Source: CAD feature listing. Evaluate the final solid. Frame: model axes, mm. A direction names the side the tool comes from. Round coordinates to 2 decimals unless told otherwise and drop trailing zeros. Loops run counter-clockwise (first coordinate to the right, second up) from the corner with the lowest first, then second, coordinate; pieces in that order, holes last. Notation, with made-up numbers: (79, 61) -> (90, 61) arc R14 ccw to (90, 71) -> close; hole circle Ø11 at (40, 89.5). An arc over 180 degrees is marked (long way). Put each result on its own line as item: value. Start each with the question number.
1. Draft query along Y for faces 4 (the cylindrical face through (-6.11, -7.46, 7.23)), 5 (the cylindrical face through (6.11, -0.31, 13.79)), 6 (the flat face through (0, -4, 1.219)). Return one class per face: pulls with the +Y half, pulls with the -Y half, needs draft (parallel to the pull), parting line crosses it, or undercut.
2. Cut plane B-B (z = 11.43). Return the cut outline in (x, y), then the cut area to 3 significant figures.
3. Cut plane D-D (z = 2). Return the cut outline in (x, y).
4. Set-up query: faces 1 (the flat face through (6.13, 7.06, 8.58)), 2 (the flat face through (6, 7.366, 4)), 3 (the cylindrical face through (5.967, -1.458, 0.724)). Return all of +Z, -Z, +X, -X, +Y, -Y with unobstructed straight access to the full face (end or side cutting, diameter ignored); none if empty.
5. Cut plane C-C (y = -3.75). Return the cut outline in (x, z), then the cut area to 3 significant figures.
6. Material intervals for L1, parallel to X at y = 2.5, z = 13; L2, parallel to Z at x = 4, y = -0.75; L3, parallel to Y at x = -6.1, z = 11.43, sorted ascending.
7. Contact query for flat-ended pins moving along their axis: pin 1 (5 mm diameter, centred on x = -2.5, y = -4, fed in from +Z); pin 2 (4 mm diameter, centred on x = -2, y = -3, fed in from +Z); pin 3 (1 mm diameter, centred on x = 6, z = 3.5, fed in from +Y). Output: stop coordinate, or through.
8. Cut plane A-A (z = 5.75). Return the cut outline in (x, y).
```python
from build123d import *

# Parameters (mm, degrees)
F1_DEPTH = 12.7
F2_R     = 2.38125
F3_DEPTH = 25.4
F5_DEPTH = 12.7


with BuildPart() as f1:
    # F0 (on Front) → F1 (new body, symmetric)
    with BuildSketch(Plane.XZ):
        with BuildLine():
            ThreePointArc((-6.731, 2.54), (-5.987051, 0.743949), (-4.191, 0))
            Line((-4.191, 0), (4.191, 0))
            ThreePointArc((4.191, 0), (5.987051, 0.743949), (6.731, 2.54))
            Line((6.731, 2.54), (6.731, 25.4))
            Line((6.731, 25.4), (5.5118, 25.4))
            Line((5.5118, 25.4), (5.5118, 2.54))
            ThreePointArc((5.5118, 2.54), (5.124947, 1.606053), (4.191, 1.2192))
            Line((4.191, 1.2192), (-4.191, 1.2192))
            ThreePointArc((-4.191, 1.2192), (-5.124947, 1.606053), (-5.5118, 2.54))
            Line((-5.5118, 2.54), (-5.5118, 25.4))
            Line((-5.5118, 25.4), (-6.731, 25.4))
            Line((-6.731, 25.4), (-6.731, 2.54))
        make_face()
    extrude(amount=F1_DEPTH, both=True)

    # F2 (on Right) → F3 (intersect, symmetric)
    with BuildSketch(Plane.YZ):
        with BuildLine():
            Line((-10.756956, 3.640789), (-8.382, 0))
            Line((-8.382, 0), (4.826, 0))
            ThreePointArc((4.826, 0), (5.572779, 1.793221), (7.366, 2.54))
            Line((7.366, 2.54), (7.366, 5.003639))
            Line((7.366, 5.003639), (4.896118, 6.262106))
            ThreePointArc((4.896118, 6.262106), (4.230106, 8.311882), (6.279882, 8.977894))
            Line((6.279882, 8.977894), (7.852802, 8.176451))
            Line((7.852802, 8.176451), (8.298947, 9.052059))
            ThreePointArc((8.298947, 9.052059), (8.373581, 9.510956), (8.167681, 9.927802))
            Line((8.167681, 9.927802), (3.468643, 14.785412))
            ThreePointArc((3.468643, 14.785412), (-2.939764, 15.257279), (-4.136388, 8.943925))
            ThreePointArc((-4.136388, 8.943925), (-7.502613, 7.201857), (-10.565319, 4.9689))
            ThreePointArc((-10.565319, 4.9689), (-10.911586, 4.340983), (-10.756956, 3.640789))
        make_face()
        with Locations((0, 11.43)):
            Circle(F2_R, mode=Mode.SUBTRACT)
    extrude(amount=F3_DEPTH, both=True, mode=Mode.INTERSECT)

    # F4 (on Top) → F5 (cut, symmetric)
    with BuildSketch(Plane.XY):
        with BuildLine():
            Line((-5.5118, 3.468643), (-5.5118, 1.640347))
            Line((-5.5118, 1.640347), (-2.670635, 0))
            Line((-2.670635, 0), (-2.413, -0.148746))
            ThreePointArc((-2.413, -0.148746), (0, -0.795307), (2.413, -0.148746))
            Line((2.413, -0.148746), (5.5118, 1.640347))
            Line((5.5118, 1.640347), (5.5118, 3.468643))
            Line((5.5118, 3.468643), (5.5118, 11.050733))
            Line((5.5118, 11.050733), (-5.5118, 11.050733))
            Line((-5.5118, 11.050733), (-5.5118, 3.468643))
        make_face()
    extrude(amount=F5_DEPTH, both=True, mode=Mode.SUBTRACT)


solid = f1.part
```
Solution:
1. face 4: pulls with the -Y half
1. face 5: undercut
1. face 6: needs draft
2. outline: (-6.73, -4.83) -> (-5.51, -4.83) -> (-5.51, -2.38) -> (-6.73, -2.38) -> close; (-6.73, 2.38) -> (-5.51, 2.38) -> (-5.51, 6.71) -> (-6.73, 6.71) -> close; (5.51, -4.83) -> (6.73, -4.83) -> (6.73, -2.38) -> (5.51, -2.38) -> close; (5.51, 2.38) -> (6.73, 2.38) -> (6.73, 6.71) -> (5.51, 6.71) -> close
2. area: 16.5 mm^2
3. outline: (-6.67, -9.69) -> (-5.4, -9.69) -> (-5.4, 1.57) -> (-5.51, 1.64) -> (-5.51, 5.81) -> (-6.67, 5.81) -> close; (5.4, -9.69) -> (6.67, -9.69) -> (6.67, 5.81) -> (5.51, 5.81) -> (5.51, 1.64) -> (5.4, 1.57) -> close
4. face 1: +X, -X
4. face 2: -Z, +X, -X, +Y
4. face 3: -Z, +X, +Y, -Y
5. outline: (-6.73, 2.54) arc R2.54 ccw to (-4.19, 0) -> (4.19, 0) arc R2.54 ccw to (6.73, 2.54) -> (6.73, 14.47) -> (5.51, 14.47) -> (5.51, 2.54) arc R1.32 cw to (4.19, 1.22) -> (-4.19, 1.22) arc R1.32 cw to (-5.51, 2.54) -> (-5.51, 14.47) -> (-6.73, 14.47) -> close
5. area: 46.7 mm^2
6. L1: x = -6.73 to -5.51, 5.51 to 6.73
6. L2: z = 0 to 1.22
6. L3: y = -4.83 to -2.38, 2.38 to 6.71
7. pin 1: stops at z = 1.5
7. pin 2: stops at z = 1.22
7. pin 3: stops at y = 7.37
8. outline: (-6.73, -9.6) -> (-5.51, -9.6) -> (-5.51, 5.9) -> (-6.73, 5.9) -> close; (5.51, -9.6) -> (6.73, -9.6) -> (6.73, 5.9) -> (5.51, 5.9) -> close
